```python
from build123d import *

# Parameters (mm, degrees)
SKETCH1_W            = 159
SKETCH1_H            = 158
BOSS_EXTRUDE1_DEPTH  = 5
SKETCH4_W            = 4
SKETCH4_H            = 158
BOSS_EXTRUDE2_DEPTH  = 35
M4_CLEARANCE_HOLE1_D = 4.5
CHAMFER2_SIZE        = 2.5


with BuildPart() as part:
    # Sketch1 → Boss-Extrude1 (new body)
    with BuildSketch(Plane(origin=(0, 0, 0), x_dir=(1, 0, 0), z_dir=(0, 1, 0))):
        with Locations((0, -79)):
            Rectangle(SKETCH1_W, SKETCH1_H)
    extrude(amount=BOSS_EXTRUDE1_DEPTH)

    # Sketch4 → Boss-Extrude2 (add)
    with BuildSketch(Plane(origin=(0, 5, 0), x_dir=(1, 0, 0), z_dir=(0, 1, 0))):
        with Locations((77.5, -79)):
            Rectangle(SKETCH4_W, SKETCH4_H)
    boss_extrude2 = extrude(amount=BOSS_EXTRUDE2_DEPTH)

    # M4 Clearance Hole1 (through all)
    with Locations(Plane.ZY.offset(-75.5)):
        with Locations((124, 20), (34, 20)):
            m4_clearance_hole1 = Hole(M4_CLEARANCE_HOLE1_D / 2)

    # Mirror2: Boss-Extrude2, M4 Clearance Hole1 across plane
    add(boss_extrude2.mirror(Plane.ZY))
    add(m4_clearance_hole1.mirror(Plane.ZY), mode=Mode.SUBTRACT)

    # Chamfer2
    chamfer2_edges = [part.edges().sort_by_distance(p)[0] for p in [
        (75.5, 5, 79),
        (-75.5, 5, 79),
    ]]
    chamfer(chamfer2_edges, length=CHAMFER2_SIZE)


solid = part.part
```
Source: CAD feature listing. Evaluate the final solid. Frame: model axes, mm. A direction names the side the tool comes from. Round coordinates to 2 decimals unless told otherwise and drop trailing zeros. Loops run counter-clockwise (first coordinate to the right, second up) from the corner with the lowest first, then second, coordinate; pieces in that order, holes last. Notation, with made-up numbers: M 36.5,-20 L 92.5,-20 A23 cw 92.5,5 Z; hole C 26,-18.75 d3. An arc over 180 degrees is marked long. Use a Markdown table: item, result. Add a question column.
1. Set-up query: faces 4 (the flat face through (-75.5, 24, 80)), 5 (the cylindrical face through (-77.528, 18.004, 32.962)). Return all of +Z, -Z, +X, -X, +Y, -Y with unobstructed straight access to the full face (end or side cutting, diameter ignored); none if empty.
2. Cut plane A-A, the plane y = 20. Output: boundary loops of the cut face in (x, z).
3. Contact query for flat-ended pins moving along their axis: pin 1 (3 mm diameter, centred on x = 54.5, z = 35, fed in from -Y); pin 2 (8 mm diameter, centred on x = 62.5, y = 12.5, fed in from +Z); pin 3 (6 mm diameter, centred on x = 20.5, z = 72.5, fed in from +Y). Output: stop coordinate, or through.
4. Cut plane C-C, the plane y = 11. Output: boundary loops of the cut face in (x, z), and give its area (3 significant figures).
5. Cut plane B-B, the plane z = 124. Output: boundary loops of the cut face in (x, y).
6. Pull-direction query (Z, two-part tool) for faces 1 (the cylindrical face through (77.53, 19.14, 121.92)), 2 (the flat face through (-1, 0, 78)), 3 (the flat face through (0, 4, 158)); classes: +Z half, -Z half, draft (parallel to the pull), parting line (faces both ways), or undercut.
7. Ray query, line 1 along Z through (x, y) = (-76.8, 20); line 2 along X through (y, z) = (23.5, 150); line 3 along Y through (x, z) = (-77.8, 124). Return the intervals inside material, ascending. Write a range as [from, to].
8. Cut plane D-D, the plane z = 66. Output: boundary loops of the cut face in (x, y), and give its area (3 significant figures).
Solution:
| question | item | result |
|---|---|---|
| 1 | face 4 | +Z, -Z, +Y |
| 1 | face 5 | +X, -X |
| 2 | outline | M -79.5,0 L -75.5,0 L -75.5,31.75 L -79.5,31.75 Z; M -79.5,36.25 L -75.5,36.25 L -75.5,121.75 L -79.5,121.75 Z; M -79.5,126.25 L -75.5,126.25 L -75.5,158 L -79.5,158 Z; M 75.5,0 L 79.5,0 L 79.5,31.75 L 75.5,31.75 Z; M 75.5,36.25 L 79.5,36.25 L 79.5,121.75 L 75.5,121.75 Z; M 75.5,126.25 L 79.5,126.25 L 79.5,158 L 75.5,158 Z |
| 3 | pin 1 | stops at y = 0 |
| 3 | pin 2 | passes through |
| 3 | pin 3 | stops at y = 5 |
| 4 | outline | M -79.5,0 L -75.5,0 L -75.5,158 L -79.5,158 Z; M 75.5,0 L 79.5,0 L 79.5,158 L 75.5,158 Z |
| 4 | area | 1,260 mm2 |
| 5 | outline | M -79.5,0 L 79.5,0 L 79.5,17.75 L 75.5,17.75 L 75.5,7.5 L 73,5 L -73,5 L -75.5,7.5 L -75.5,17.75 L -79.5,17.75 Z; M -79.5,22.25 L -75.5,22.25 L -75.5,40 L -79.5,40 Z; M 75.5,22.25 L 79.5,22.25 L 79.5,40 L 75.5,40 Z |
| 6 | face 1 | undercut |
| 6 | face 2 | draft |
| 6 | face 3 | +Z half |
| 7 | line 1 | z = [0, 31.75], [36.25, 121.75], [126.25, 158] |
| 7 | line 2 | x = [-79.5, -75.5], [75.5, 79.5] |
| 7 | line 3 | y = [0, 17.75], [22.25, 40] |
| 8 | outline | M -79.5,0 L 79.5,0 L 79.5,40 L 75.5,40 L 75.5,7.5 L 73,5 L -73,5 L -75.5,7.5 L -75.5,40 L -79.5,40 Z |
| 8 | area | 1,080 mm2 |
